Part model, mm, in its own coordinate system. A direction names the side the tool comes from. Coordinates: 2 decimals unless noted, no trailing zeros. Write each loop counter-clockwise with the first axis right and the second up, starting at its lowest first coordinate (ties: lowest second). Pieces come first, ordered by that corner, then holes. Notation, with made-up numbers: (53, 67.5) -> (59, 67.5) arc R20 ccw to (59, 81.5) -> close; hole circle Ø9 at (35.25, -38). An arc over 180 degrees is marked (long way). Write item = value, one per line. Start each with the question number.
Q1. Pull direction X, two halves, no side cores. Call faces 4 (the flat face through (8, 6.35, 6)), 5 (the flat face through (-31.75, -16, 0)), 6 (the cylindrical face through (-7.559, -6.528, -5.796)): released by +X, released by -X, zero draft, split by the parting line, or undercut.
Q2. Tool access for faces 1 (the flat face through (-29, -12.7, 0)), 2 (the flat face through (29, 0, 0)), 3 (the cylindrical face through (21.199, -19.833, 6.676)): list every direction of +Z, -Z, +X, -X, +Y, -Y with a clear straight run to the whole face (end or side of a thin tool).
Q3. Pin check, flat tips, straight feed: P1, Ø5, axis at x = -28, z = 2.5, coming from the -Y side; P2, Ø5, axis at y = -9.5, z = -13.5, coming from the -X side; P3, Ø11.5, axis at x = 0, z = 0, coming from the +Y side; P4, Ø15, axis at x = 3.5, z = 0, coming from the +Y side. Stop position of each tip, or through.
Q4. Band-saw the part on C-C, the plane y = -1. List the corners of the cut face in (x, z) (3 decimals).
Q5. Band-saw the part on D-D, the plane y = -13.75. List the corners of the cut face in (x, z) (3 decimals), plus the area to 3 significant figures.
Q6. Probe line 1 (Z direction, x = 0, y = -6.25) (3 decimals); line 2 (Y direction, x = -27, z = 0.5); line 3 (X direction, y = -0.5, z = -0.5). List the from-to ranges inside material, lowest first.
from build123d import *

# Parameters (mm, degrees)
F0_W     = 50.8
F0_H     = 50.8
F1_DEPTH = 12.7
F2_W     = 6.35
F2_H     = 50.8
F2_W_2   = 50.8
F3_DEPTH = 6.35
F4_W     = 6.35
F4_H     = 50.8
F4_W_2   = 50.8
F5_DEPTH = 6.35
F6_R     = 9.525
F7_DEPTH = 38.1
F8_R     = 22.225
F8_R_2   = 9.525
F9_DEPTH = 1.5875


# Not quite as in the source:
# - a feature names something its author has since deleted; it is built from what else it names


with BuildPart() as f1:
    # F0 (on Front) → F1 (new body)
    with BuildSketch(Plane.XZ):
        Rectangle(F0_W, F0_H)
    extrude(amount=F1_DEPTH)

    # F2 (on face) → F3 (join)
    with BuildSketch(Plane.XZ.offset(12.7)):
        with Locations((-28.575, 0)):
            Rectangle(F2_W, F2_H)
        Rectangle(F2_W_2, F2_H)
        with Locations((28.575, 0)):
            Rectangle(F2_W, F2_H)
    extrude(amount=F3_DEPTH)

    # F4 (on face) → F5 (join)
    with BuildSketch(Plane(origin=(0, 0, 0), x_dir=(-1, 0, 0), z_dir=(0, 1, 0))):
        with Locations((28.575, 0)):
            Rectangle(F4_W, F4_H)
        Rectangle(F4_W_2, F4_H)
        with Locations((-28.575, 0)):
            Rectangle(F4_W, F4_H)
    extrude(amount=F5_DEPTH)

    # F6 (on face) → F7 (cut)
    with BuildSketch(Plane.XZ.offset(19.05)):
        Circle(F6_R)
    extrude(amount=-F7_DEPTH, mode=Mode.SUBTRACT)

    # F8 (on face) → F9 (join)
    with BuildSketch(Plane.XZ.offset(19.05)):
        Circle(F8_R)
        Circle(F8_R_2, mode=Mode.SUBTRACT)
        Circle(F8_R_2)
    extrude(amount=F9_DEPTH)


solid = f1.part
Ans:
q1.face_4 = zero draft
q1.face_5 = released by -X
q1.face_6 = undercut
q2.face_1 = +Z, -Z, -X
q2.face_2 = +Z, -Z, +X
q2.face_3 = -Y
q3.P1 = -19.05
q3.P2 = -25.4
q3.P3 = -19.05
q3.P4 = 6.35
q4.outline = (-25.4, -25.4) -> (25.4, -25.4) -> (25.4, 25.4) -> (-25.4, 25.4) -> close; hole circle Ø19.05 at (0, 0)
q5.outline = (-31.75, -25.4) -> (31.75, -25.4) -> (31.75, 25.4) -> (-31.75, 25.4) -> close; hole circle Ø19.05 at (0, 0)
q5.area = 2,940 mm2
q6.line_1 = -25.4 to -9.525, 9.525 to 25.4
q6.line_2 = -19.05 to -12.7, 0 to 6.35
q6.line_3 = -25.4 to -9.51, 9.51 to 25.4
